Design review of the part built by this model. Coordinates are the model's own, in mm. Face numbers are marked on the shaded views. Round coordinates to 2 decimals unless told otherwise and drop trailing zeros. Order: outer loops, then holes, each group sorted by start corner. A loop starts at its lowest first (then second) coordinate and runs counter-clockwise, first axis right, second up. Notation, with made-up numbers: (30, -18) - (53, -18) arc R22 cw to (53, 4) - close; hole circle Ø6 at (87.5, -6). An arc over 180 degrees is marked (long way). Use CSV: the item, a comma, the result in double quotes.
from build123d import *
from build123d.topology import SkipClean

# Parameters (mm, degrees)
SKETCH1_W           = 5
SKETCH1_H           = 53.385
CHAMFER1_SIZE       = 2
SHELL1_T            = -0.25
CUT_EXTRUDE1_DEPTH  = 10
BOSS_EXTRUDE1_DEPTH = 5
CUT_EXTRUDE2_DEPTH  = 76.663177636
CIRPATTERN1_COUNT   = 30


with BuildPart() as part:
    # Sketch1 → Revolve1 (revolve)
    with BuildSketch(Plane.YZ, mode=Mode.PRIVATE) as revolve1_sk:
        with Locations((2.5, 26.6925)):
            Rectangle(SKETCH1_W, SKETCH1_H)
    revolve(revolve1_sk.sketch.rotate(Axis((0, -14.724137931, 0), (0, 1, 0)), 180), axis=Axis((0, -14.724137931, 0), (0, 1, 0)))

    # Chamfer1
    chamfer1_edges = [part.edges().sort_by_distance(p)[0] for p in [
        (0, 0, 53.385),
    ]]
    chamfer(chamfer1_edges, length=CHAMFER1_SIZE)

    # Shell1
    shell1_openings = [part.faces().sort_by_distance(p)[0] for p in [
        (0, 5, 0),
    ]]
    offset(amount=SHELL1_T, openings=shell1_openings, kind=Kind.INTERSECTION)

    # Sketch2 → Cut-Extrude1 (cut)
    with BuildSketch(Plane.XZ):
        with BuildLine():
            ThreePointArc((-29.385, 0), (0, -29.385), (29.385, 0))
            Line((29.385, 0), (-29.385, 0))
        make_face()
        with BuildLine():
            Line((-29.385, 0), (29.385, 0))
            ThreePointArc((29.385, 0), (0, 29.385), (-29.385, 0))
        make_face()
    extrude(amount=-CUT_EXTRUDE1_DEPTH, mode=Mode.SUBTRACT)

    # Sketch2<3> → Boss-Extrude1 (add)
    with BuildSketch(Plane.XZ):
        with BuildLine():
            ThreePointArc((-29.385, 0), (0, 29.385), (29.385, 0))
            Line((29.385, 0), (31.385, 0))
            ThreePointArc((31.385, 0), (0, 31.385), (-31.385, 0))
            Line((-31.385, 0), (-29.385, 0))
        make_face()
        with BuildLine():
            Line((31.385, 0), (29.385, 0))
            ThreePointArc((29.385, 0), (0, -29.385), (-29.385, 0))
            Line((-29.385, 0), (-31.385, 0))
            ThreePointArc((-31.385, 0), (0, -31.385), (31.385, 0))
        make_face()
    extrude(amount=-BOSS_EXTRUDE1_DEPTH)

    # Sketch2<4> → Cut-Extrude2 (cut, symmetric)
    with SkipClean():  # the faces are left unmerged after this step: merging them gives an invalid solid
        with BuildSketch(Plane.XZ):
            with BuildLine():
                ThreePointArc((-45.38, 0), (-41.38, -4), (-37.38, 0))
                Line((-37.38, 0), (-45.38, 0))
            make_face()
            with BuildLine():
                Line((-45.38, 0), (-37.38, 0))
                ThreePointArc((-37.38, 0), (-41.38, 4), (-45.38, 0))
            make_face()
        cut_extrude2 = extrude(amount=CUT_EXTRUDE2_DEPTH, both=True, mode=Mode.SUBTRACT)

    # CirPattern1: Cut-Extrude2 ×30 about axis
    with SkipClean():  # the faces are left unmerged after this step: merging them gives an invalid solid
        cirpattern1_axis = Axis((0, 0, 0), (0, 1, 0))
        for i in range(1, CIRPATTERN1_COUNT):
            add(cut_extrude2.rotate(cirpattern1_axis, i * 360 / CIRPATTERN1_COUNT), mode=Mode.SUBTRACT)


solid = part.part
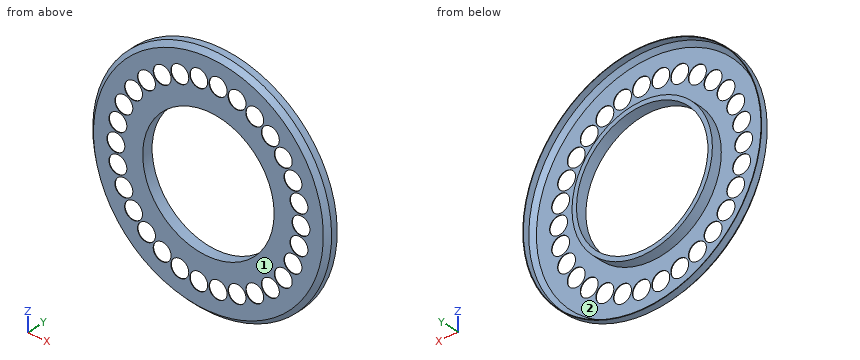
1) Insertion check: pin 1 Ø9 at (x, z) = (-37.8, 16.83) entering from +Y; pin 2 Ø7 at (x, z) = (40.48, 8.6) entering from -Y; pin 3 Ø1.5 at (x, y) = (-3.5, 4) entering from -Z. Each pin has a flat end and moves straight along its axis. Give the tip position at first contact, or say it passes through.
Data:
pin 1,"stops at y = 0.25"
pin 2,"passes through"
pin 3,"stops at z = -53.31"
2) We need section B-B (x = 14). Give the number of separate pieces and of enclosed holes in the cut face, then the cut area to 3 significant figures.
Data:
separate pieces,"4"
enclosed holes,"0"
area,"32.3 mm2"
3) We need section A-A (z = 0). Give the boundary of the cut face in (x, y) (3 decimals), then the cut area to 3 significant figures.
Data:
outline,"(-53.385, 2) - (-51.385, 0) - (-45.38, 0) - (-45.38, 0.25) - (-51.281, 0.25) - (-53.135, 2.104) - (-53.135, 5) - (-53.385, 5) - close; (-37.38, 0) - (-29.385, 0) - (-29.385, 5) - (-31.385, 5) - (-31.385, 0.25) - (-37.38, 0.25) - close; (29.385, 0) - (37.38, 0) - (37.38, 0.25) - (31.385, 0.25) - (31.385, 5) - (29.385, 5) - close; (45.38, 0) - (51.385, 0) - (53.385, 2) - (53.385, 5) - (53.135, 5) - (53.135, 2.104) - (51.281, 0.25) - (45.38, 0.25) - close"
area,"28.8 mm2"
4) The part is to be moulded in two halves that separate along Z. For the marked faces 1 and 2, say which applies: +Z half, -Z half, draft (parallel to the pull), parting line (faces both ways), or undercut.
Data:
face 1,"draft"
face 2,"undercut"
5) To check wall thickness, follow L1, parallel to Z at x = 24.5, y = 2; L2, parallel to Z at x = 19, y = 2.7; L3, parallel to Z at x = 38, y = 3.7. State the ranges of each line that lie inside material, in increasing order. Write a range as from..to.
Data:
L1,"z = -47.43..-47.03, -19.62..-16.22, 16.22..19.62, 47.03..47.43"
L2,"z = -49.89..-49.62, -24.98..-22.42, 22.42..24.98, 49.62..49.89"
L3,"z = -37.5..-37.14, 37.14..37.5"
